Verification items for the finished model (mm, model axes). A direction names the side the tool comes from. Coordinates: 2 decimals unless noted, no trailing zeros. Write each loop counter-clockwise with the first axis right and the second up, starting at its lowest first coordinate (ties: lowest second). Pieces come first, ordered by that corner, then holes. Notation, with made-up numbers: (-10, -4) -> (43, -4) arc R15 cw to (43, 13) -> close; hole circle Ø11 at (-30.75, 75). An arc over 180 degrees is marked (long way). Write item = value, one per line. Start each with the question number.
(1) Section check D-D (z = 13). Record the cut outline in (x, y) (3 decimals), plus the area to 3 significant figures.
(2) Mould release check, pull along X, two halves, no side actions. Record for faces 4 (the face through (0, -4.762, 2)), 5 (the face through (-11.11, -0.1, 1.61)), 6 (the face through (0, -22.225, 27)), 7 (the face through (-18.256, 0, 19)): released by +X, released by -X, zero draft, split by the parting line, or undercut.
(3) Material ranges on probe 1 along Y at (x, z) = (3, 36) (3 decimals); probe 2 along X at (y, z) = (-8, 1) (1 decimal), recorded low to high. Write a range as [from, to].
(4) Set-up check for faces 1 (the face through (-21.431, 0, 19)), 2 (the face through (5.487, -17.239, 5.085)), 3 (the face through (-20, 0, 34.925)): record each of +Z, -Z, +X, -X, +Y, -Y from which the full face is reachable in a straight line by a thin tool's end or side.
(5) Gauge pin test, flat ends, axial feed: pin 1 Ø2 at (x, y) = (7.5, -14.5) entering from -Z; pin 2 Ø12.5 at (x, y) = (11.5, 3) entering from +Z (3 decimals); pin 3 Ø8 at (x, y) = (-24.5, -6) entering from +Z (3 decimals); pin 4 Ø16 at (y, z) = (5, 16.5) entering from -X. Record the tip position at first contact, or that the pin passes through.
(6) Section check A-A (x = -13.5). Record the cut outline in (y, z) (3 decimals).
(7) Section check B-B (y = 8.5). Record the cut outline in (x, z) (3 decimals).
(8) Section check C-C (y = 0). Record the cut outline in (x, z) (1 decimal), plus the area to 3 significant figures.
```python
from build123d import *

# Parameters (mm, degrees)
SKETCH1_W            = 57.15
SKETCH1_H            = 38.1
BOSS_EXTRUDE1_DEPTH  = 3.175
SKETCH2_R            = 2
CUT_EXTRUDE1_DEPTH   = 35.48932806
BOSS_EXTRUDE2_START  = -3.175
SKETCH3_W            = 57.15
SKETCH3_H            = 3.175
BOSS_EXTRUDE2_DEPTH  = 53.975
CUT_EXTRUDE2_REACH   = 73.982
SKETCH5_R            = 2
FILLET1_R            = 6.35
FILLET1_OF_MIRROR1_R = 6.35
RIB1_REACH           = 77.839
SKETCH7_WALL_W       = 191.77895835
SKETCH7_WALL_H       = 3.175


with BuildPart() as part:
    # Sketch1 → Boss-Extrude1 (new body)
    with BuildSketch(Plane.XY):
        Rectangle(SKETCH1_W, SKETCH1_H)
    extrude(amount=BOSS_EXTRUDE1_DEPTH)

    # Sketch2 → Cut-Extrude1 (cut, through all)
    with BuildSketch(Plane.XY.offset(3.175)):
        with Locations((-13.5, 8.5)):
            Circle(SKETCH2_R)
        with Locations((13.5, 8.5)):
            Circle(SKETCH2_R)
        with Locations((13.5, -8.5)):
            Circle(SKETCH2_R)
        with Locations((-13.5, -8.5)):
            Circle(SKETCH2_R)
        with BuildLine():
            Line((-6.35, 4.7625), (6.35, 4.7625))
            ThreePointArc((6.35, 4.7625), (11.1125, 0), (6.35, -4.7625))
            Line((6.35, -4.7625), (-6.35, -4.7625))
            ThreePointArc((-6.35, -4.7625), (-11.1125, 0), (-6.35, 4.7625))
        make_face()
    extrude(amount=-CUT_EXTRUDE1_DEPTH, mode=Mode.SUBTRACT)

    # Sketch3 → Boss-Extrude2 (add)
    with BuildSketch(Plane.XY.offset(3.175).offset(BOSS_EXTRUDE2_START)):
        with Locations((0, 20.6375)):
            Rectangle(SKETCH3_W, SKETCH3_H)
    boss_extrude2 = extrude(amount=BOSS_EXTRUDE2_DEPTH)

    # Sketch5 → Cut-Extrude2 (cut, up to next)
    with BuildSketch(Plane.XZ.offset(-19.05), mode=Mode.PRIVATE) as cut_extrude2_sk1:
        with Locations((-22.225, 47.625)):
            Circle(SKETCH5_R)
    cut_extrude2_tool1 = extrude(cut_extrude2_sk1.sketch, amount=-CUT_EXTRUDE2_REACH, mode=Mode.PRIVATE) & part.part
    # Sketch5 → Cut-Extrude2 (cut, up to next)
    with BuildSketch(Plane.XZ.offset(-19.05), mode=Mode.PRIVATE) as cut_extrude2_sk2:
        with Locations((22.225, 47.625)):
            Circle(SKETCH5_R)
    cut_extrude2_tool2 = extrude(cut_extrude2_sk2.sketch, amount=-CUT_EXTRUDE2_REACH, mode=Mode.PRIVATE) & part.part
    cut_extrude2_1 = cut_extrude2_tool1.solids().sort_by_distance((-22.225, 19.05, 47.625))[0]
    add(cut_extrude2_1, mode=Mode.SUBTRACT)
    cut_extrude2_2 = cut_extrude2_tool2.solids().sort_by_distance((22.225, 19.05, 47.625))[0]
    add(cut_extrude2_2, mode=Mode.SUBTRACT)
    cut_extrude2 = cut_extrude2_1 + cut_extrude2_2  # Cut-Extrude2 as one shape, for the pattern or mirror that repeats it

    # Fillet1
    fillet1_edges = [part.edges().sort_by_distance(p)[0] for p in [
        (28.575, 20.6375, 53.975),
        (-28.575, 20.6375, 53.975),
        (0, 19.05, 3.175),
    ]]
    fillet(fillet1_edges, radius=FILLET1_R)

    # Mirror1: Boss-Extrude2, Cut-Extrude2 across plane
    add(boss_extrude2.mirror(Plane.ZX))
    add(cut_extrude2.mirror(Plane.ZX), mode=Mode.SUBTRACT)

    # Fillet1 of Mirror1
    fillet1_of_mirror1_edges = [part.edges().sort_by_distance(p)[0] for p in [
        (28.575, -20.6375, 53.975),
        (-28.575, -20.6375, 53.975),
        (0, -19.05, 3.175),
    ]]
    fillet(fillet1_of_mirror1_edges, radius=FILLET1_OF_MIRROR1_R)

    # Sketch7 wall → Rib1 (add, up to next)
    with BuildSketch(Plane(origin=(-19.84375, 0, 34.925), x_dir=(0, -1, 0), z_dir=(0, 0, 1)), mode=Mode.PRIVATE) as rib1_sk1:
        Rectangle(SKETCH7_WALL_W, SKETCH7_WALL_H)
    rib1_tool1 = extrude(rib1_sk1.sketch, amount=-RIB1_REACH, mode=Mode.PRIVATE) - part.part
    add(rib1_tool1.solids().sort_by_distance((-19.84375, 0, 34.925))[0])


solid = part.part
```
Response:
q1.outline = (-28.575, -22.225) -> (28.575, -22.225) -> (28.575, -19.05) -> (-18.256, -19.05) -> (-18.256, 19.05) -> (28.575, 19.05) -> (28.575, 22.225) -> (-28.575, 22.225) -> (-28.575, 19.05) -> (-21.431, 19.05) -> (-21.431, -19.05) -> (-28.575, -19.05) -> close
q1.area = 484 mm2
q2.face_4 = undercut
q2.face_5 = undercut
q2.face_6 = zero draft
q2.face_7 = released by +X
q3.probe_1 = [-22.225, -19.05], [19.05, 22.225]
q3.probe_2 = [-28.6, -15.4], [-11.6, 11.6], [15.4, 28.6]
q4.face_1 = +Z, -X
q4.face_2 = +Z, +X
q4.face_3 = +Z, +X, -X
q5.pin_1 = 0
q5.pin_2 = 3.175
q5.pin_3 = 34.925
q5.pin_4 = -21.43
q6.outline = (-22.225, 0) -> (-10.5, 0) -> (-10.5, 3.175) -> (-12.7, 3.175) arc R6.35 cw to (-19.05, 9.525) -> (-19.05, 53.975) -> (-22.225, 53.975) -> close; (-6.5, 0) -> (6.5, 0) -> (6.5, 3.175) -> (-6.5, 3.175) -> close; (10.5, 0) -> (22.225, 0) -> (22.225, 53.975) -> (19.05, 53.975) -> (19.05, 9.525) arc R6.35 cw to (12.7, 3.175) -> (10.5, 3.175) -> close
q7.outline = (-28.575, 0) -> (-15.5, 0) -> (-15.5, 3.175) -> (-18.256, 3.175) -> (-18.256, 34.925) -> (-21.431, 34.925) -> (-21.431, 3.175) -> (-28.575, 3.175) -> close; (-11.5, 0) -> (11.5, 0) -> (11.5, 3.175) -> (-11.5, 3.175) -> close; (15.5, 0) -> (28.575, 0) -> (28.575, 3.175) -> (15.5, 3.175) -> close
q8.outline = (-28.6, 0) -> (-11.1, 0) -> (-11.1, 3.2) -> (-18.3, 3.2) -> (-18.3, 34.9) -> (-21.4, 34.9) -> (-21.4, 3.2) -> (-28.6, 3.2) -> close; (11.1, 0) -> (28.6, 0) -> (28.6, 3.2) -> (11.1, 3.2) -> close
q8.area = 212 mm2
